CAD build for the part. Positions are in the model's coordinates, mm. Give positions to 0.01 mm unless a question says otherwise; leave off trailing zeros. Loops run counter-clockwise (first coordinate to the right, second up) from the corner with the lowest first, then second, coordinate; pieces in that order, holes last. Notation, with made-up numbers: M 70.5,76.25 L 118.5,76.25 A4 ccw 118.5,82.25 Z; hole C 6.5,81 d11. An arc over 180 degrees is marked long. One line per question, with ' | ' between items.
```python
from build123d import *

# Parameters (mm, degrees)
F0_R     = 1.5
F0_R_2   = 18
F1_DEPTH = 60
F2_R     = 5


with BuildPart() as f1:
    # F0 (on Top) → F1 (new body)
    with BuildSketch(Plane.XY):
        with BuildLine():
            ThreePointArc((-14.1902170115, 12.6347829885), (-13.4350288425, 13.4350288425), (-12.6347829885, 14.1902170115))
            ThreePointArc((-12.6347829885, 14.1902170115), (-12.533925941, 14.5895383872), (-12.5, 15))
            ThreePointArc((-12.5, 15), (-17.0340178799, 16.4535375002), (-14.1902170115, 12.6347829885))
        make_face()
        with Locations((-15, 15)):
            Circle(F0_R, mode=Mode.SUBTRACT)
        with BuildLine():
            ThreePointArc((12.6347829885, 14.1902170115), (13.232233047, 13.232233047), (14.1902170115, 12.6347829885))
            ThreePointArc((14.1902170115, 12.6347829885), (13.4350288425, 13.4350288425), (12.6347829885, 14.1902170115))
        make_face()
        with BuildLine():
            ThreePointArc((12.6347829885, 14.1902170115), (13.4350288425, 13.4350288425), (14.1902170115, 12.6347829885))
            ThreePointArc((14.1902170115, 12.6347829885), (16.4535375002, 12.9659821201), (17.5, 15))
            ThreePointArc((17.5, 15), (14.5895383872, 17.466074059), (12.6347829885, 14.1902170115))
        make_face()
        with Locations((15, 15)):
            Circle(F0_R, mode=Mode.SUBTRACT)
        with BuildLine():
            ThreePointArc((12.6347829885, -14.1902170115), (13.4350288425, -13.4350288425), (14.1902170115, -12.6347829885))
            ThreePointArc((14.1902170115, -12.6347829885), (13.232233047, -13.232233047), (12.6347829885, -14.1902170115))
        make_face()
        with BuildLine():
            ThreePointArc((17.5, -15), (16.4535375002, -12.9659821201), (14.1902170115, -12.6347829885))
            ThreePointArc((14.1902170115, -12.6347829885), (13.4350288425, -13.4350288425), (12.6347829885, -14.1902170115))
            ThreePointArc((12.6347829885, -14.1902170115), (14.5895383872, -17.466074059), (17.5, -15))
        make_face()
        with Locations((15, -15)):
            Circle(F0_R, mode=Mode.SUBTRACT)
        with BuildLine():
            ThreePointArc((-14.1902170115, -12.6347829885), (-13.4350288425, -13.4350288425), (-12.6347829885, -14.1902170115))
            ThreePointArc((-12.6347829885, -14.1902170115), (-13.232233047, -13.232233047), (-14.1902170115, -12.6347829885))
        make_face()
        with BuildLine():
            ThreePointArc((-12.5, -15), (-12.533925941, -14.5895383872), (-12.6347829885, -14.1902170115))
            ThreePointArc((-12.6347829885, -14.1902170115), (-13.4350288425, -13.4350288425), (-14.1902170115, -12.6347829885))
            ThreePointArc((-14.1902170115, -12.6347829885), (-17.0340178799, -16.4535375002), (-12.5, -15))
        make_face()
        with Locations((-15, -15)):
            Circle(F0_R, mode=Mode.SUBTRACT)
        with BuildLine():
            ThreePointArc((14.1902170115, -12.6347829885), (17.7568877231, -6.7596551976), (19, 0))
            ThreePointArc((19, 0), (17.7568877231, 6.7596551976), (14.1902170115, 12.6347829885))
            ThreePointArc((14.1902170115, 12.6347829885), (13.232233047, 13.232233047), (12.6347829885, 14.1902170115))
            ThreePointArc((12.6347829885, 14.1902170115), (0, 19), (-12.6347829885, 14.1902170115))
            ThreePointArc((-12.6347829885, 14.1902170115), (-13.232233047, 13.232233047), (-14.1902170115, 12.6347829885))
            ThreePointArc((-14.1902170115, 12.6347829885), (-19, 0), (-14.1902170115, -12.6347829885))
            ThreePointArc((-14.1902170115, -12.6347829885), (-13.232233047, -13.232233047), (-12.6347829885, -14.1902170115))
            ThreePointArc((-12.6347829885, -14.1902170115), (0, -19), (12.6347829885, -14.1902170115))
            ThreePointArc((12.6347829885, -14.1902170115), (13.232233047, -13.232233047), (14.1902170115, -12.6347829885))
        make_face()
        Circle(F0_R_2, mode=Mode.SUBTRACT)
        with BuildLine():
            ThreePointArc((-14.1902170115, 12.6347829885), (-13.232233047, 13.232233047), (-12.6347829885, 14.1902170115))
            ThreePointArc((-12.6347829885, 14.1902170115), (-13.4350288425, 13.4350288425), (-14.1902170115, 12.6347829885))
        make_face()
    extrude(amount=-F1_DEPTH)

    # F2
    f2_edges = [f1.edges().sort_by_distance(p)[0] for p in [
        (-14.190217, 12.634783, -30),
        (-14.190217, -12.634783, -30),
        (12.634783, 14.190217, -30),
        (-12.634783, 14.190217, -30),
        (14.190217, 12.634783, -30),
        (14.190217, -12.634783, -30),
        (12.634783, -14.190217, -30),
        (-12.634783, -14.190217, -30),
    ]]
    fillet(f2_edges, radius=F2_R)


solid = f1.part
```
Item 1: Saw through at D-D on z = -29.5. State how many separate pieces and enclosed holes the cut face has, and give its area (3 significant figures).
Conclusion:
separate pieces: 1 | enclosed holes: 5 | area: 191 mm²
Item 2: Drop flat-ended pins along their axis: P1, Ø1.5, axis at x = 6, z = -37, coming from the -Y side; P2, Ø5, axis at x = 5, z = -51.5, coming from the +Y side; P3, Ø12, axis at x = 14, z = -22.5, coming from the -Y side. Give the stop position or say it passes through.
Conclusion:
P1: y = -18.26 | P2: y = 18.83 | P3: y = -17.5
Item 3: Saw through at B-B on y = 6. Give the cut face in (x, z).
Conclusion:
outline: M -18.03,-60 L -16.97,-60 L -16.97,0 L -18.03,0 Z; M 16.97,-60 L 18.03,-60 L 18.03,0 L 16.97,0 Z
Item 4: Saw through at C-C on x = 15. Give the cut face in (y, z), and give its area (3 significant figures).
Conclusion:
outline: M -17.5,-60 L -16.5,-60 L -16.5,0 L -17.5,0 Z; M -13.5,-60 L -9.95,-60 L -9.95,0 L -13.5,0 Z; M 9.95,-60 L 13.5,-60 L 13.5,0 L 9.95,0 Z; M 16.5,-60 L 17.5,-60 L 17.5,0 L 16.5,0 Z | area: 546 mm²
Item 5: Drill centre lines: line 1 along Y through (x, z) = (-15, -23); line 2 along Y through (x, z) = (-16, -38); line 3 along Y through (x, z) = (-0.5, -3.5). Where is each one in solid material? Low to high. Write a range as [from, to].
Conclusion:
line 1: [-17.5, -16.5], [-13.5, -9.95], [9.95, 13.5], [16.5, 17.5] | line 2: [-17.29, -16.12], [-13.88, -8.25], [8.25, 13.88], [16.12, 17.29] | line 3: [-18.99, -17.99], [17.99, 18.99]
Item 6: Saw through at A-A on x = 0. Give the cut face in (y, z), and give its area (3 significant figures).
Conclusion:
outline: M -19,-60 L -18,-60 L -18,0 L -19,0 Z; M 18,-60 L 19,-60 L 19,0 L 18,0 Z | area: 120 mm²
